Read the model definition and answer for the solid it produces. Units are mm, in the model's axes. A direction names the side the tool comes from. Coordinates: 2 decimals unless noted, no trailing zeros. Write each loop counter-clockwise with the first axis right and the second up, starting at its lowest first coordinate (ties: lowest second). Pieces come first, ordered by that corner, then holes. Notation, with made-up numbers: (76, 18.25) -> (100, 18.25) arc R31 ccw to (100, 56.25) -> close; hole circle Ø2 at (38.5, 15). An arc over 180 degrees is marked (long way). Use CSV: the item, a comma, the result in double quotes.
Autodesk Inventor part; units mm, degrees
ref_plane "YZ Plane" through (0, 0, 0) normal (1, 0, 0) x (0, 1, 0)
ref_plane "XZ Plane" through (0, 0, 0) normal (0, 1, 0) x (-1, 0, 0)
ref_plane "XY Plane" through (0, 0, 0) normal (0, 0, 1) x (1, 0, 0)
sketch "Sketch1" plane through (0, 0, 0) normal (0, 0, 1) x (1, 0, 0)
  line L0 (0, 0) -> (70, 0)
  line L1 (70, 0) -> (70, 77.5)
  line L2 (70, 77.5) -> (0, 77.5)
  line L3 (0, 77.5) -> (0, 0)
  dimension "d0" = 70
  dimension "d1" = 77.5
extrude "Extrusion1" add sketch "Sketch1" along normal blind 70
sketch "Sketch3" plane through (0, 0, 70) normal (0, 0, 1) x (1, 0, 0)
  line L0 (0, 0) -> (70, 0)
  line L1 (70, 77.5) -> (0, 77.5)
  line L2 (70, 0) -> (35, 0)
  line L3 (35, 0) -> (35, 77.5)
  line L4 (35, 77.5) -> (70, 77.5)
  line L5 (70, 77.5) -> (70, 0)
extrude "Extrusion3" cut sketch "Sketch3" against normal through all
sketch "Sketch4" plane through (0, 77.5, 70) normal (0, 1, 0) x (1, 0, 0)
  line L0 (0, 70) -> (0, 0)
  line L1 (0, 0) -> (-12.5, 0)
  line L2 (35, 70) -> (0, 70)
  arc A0 (-12.5, 0) -> (0, 70) centre (-1137.8005, 237.0626) ccw
  line L3 (-12.5, -10) -> (35, -10) construction
  dimension "d9" = 1150
  dimension "d54" = 47.5
  dimension "d55" = 10
extrude "Extrusion4" add sketch "Sketch4" against normal blind 77.5
sketch "Sketch5" plane through (35, 0, 70) normal (1, 0, 0) x (0, 0, -1)
  line L0 (0, 77.5) -> (0, 86.25)
  line L1 (0, 0) -> (0, -8.75)
  line L2 (0, 0) -> (0, 77.5)
  line L3 (70, 77.5) -> (70, 0)
  arc A0 (0, 86.25) -> (70, 77.5) centre (177.5728, 1222.4577) ccw
  arc A1 (70, 0) -> (0, -8.75) centre (177.5728, -1144.9577) ccw
  line L4 (0, 77.5) -> (70, 77.5)
  line L5 (70, 0) -> (0, 0)
  line L6 (-10, 86.25) -> (-10, -8.75) construction
  point P0 (-10, 38.75)
  point P1 (0, 38.75)
  dimension "d14" = 1150
  dimension "d15" = 1150
  dimension "d52" = 10
  dimension "d53" = 95
extrude "Extrusion5" add sketch "Sketch5" against normal blind 55 contours L0 A0 L4 | L5 A1 L1
sketch "Sketch6" plane through (-20, 0, 0) normal (0, 1, 0) x (1, 0, 0)
  line L0 (20, 0) -> (0, 0)
  line L1 (0, -70) -> (0, 0)
  arc A0 (7.5, -70) -> (20, 0) centre (-1117.8005, 167.0626) ccw
  line L2 (7.5, -70) -> (0, -70)
extrude "Extrusion6" cut sketch "Sketch6" along normal through all both and the other way through all
fillet "Fillet3" radius 19.35 2 edges at (-5.7463, 81.368, 35.3063) (-5.7463, -3.868, 35.3063)
sketch "Sketch8" plane through (0, 0, 70) normal (0, 0, 1) x (1, 0, 0)
  line L0 (35, 86.25) -> (35, -8.75)
  line L1 (35, 77.5) -> (35, 0)
  circle A0 centre (35, 38.75) radius 35
  point P0 (0, 0)
  dimension "d23" = 70
extrude "Extrusion7" cut sketch "Sketch8" against normal blind 17.5
sketch "Sketch17" plane through (35, 0, 0) normal (1, 0, 0) x (0, 0, -1)
  line L0 (-5, 13.75) -> (-40, 13.75)
  line L1 (-40, 13.75) -> (-40, 63.75)
  line L2 (-40, 63.75) -> (-5, 63.75)
  line L3 (-5, 63.75) -> (-5, 13.75)
  line L4 (0, 77.5) -> (0, 0)
  line L5 (-70, 86.25) -> (-70, 73.75)
  arc A0 (-70, 86.25) -> (0, 77.5) centre (107.5728, 1222.4577) ccw
  line L6 (-70, 3.75) -> (-70, 73.75)
  line L7 (-70, 3.75) -> (-70, -8.75)
  arc A1 (0, 0) -> (-70, -8.75) centre (107.5728, -1144.9577) ccw
  point P0 (-5, 38.75)
  point P1 (0, 38.75)
  dimension "d62" = 35
  dimension "d63" = 50
  dimension "d77" = 5
extrude "Extrusion15" cut sketch "Sketch17" against normal through all
sketch "Sketch21" plane through (35, 13.75, 5) normal (1, 0, 0) x (0, 0, -1)
  line L0 (-8, 5) -> (0, 5)
  line L1 (0, 5) -> (0, 45)
  line L2 (0, 45) -> (-8, 45)
  line L3 (-8, 45) -> (-8, 5)
  line L4 (0, 0) -> (0, 50)
  point P0 (5, -13.75)
  point P1 (-35, 25)
  point P2 (0, 25)
  dimension "d78" = 40
  dimension "d79" = 8
extrude "Extrusion19" cut sketch "Sketch21" against normal blind 30
sketch "Sketch22" plane through (35, 63.75, 40) normal (0, 1, 0) x (1, 0, 0)
  line L0 (0, 35) -> (0, 0)
  circle A0 centre (-15, 15) radius 2.5
  line L1 (0, 35) -> (-35.1041, 35)
  point P0 (-35, 40)
  dimension "d82" = 5
  dimension "d90" = 20
  dimension "d91" = 15
extrude "Extrusion20" cut sketch "Sketch22" against normal through all
sketch "Sketch23" plane through (35, 13.75, 40) normal (1, 0, 0) x (0, 0, -1)
  line L0 (35, 5) -> (27, 5) construction
  line L1 (27, 5) -> (27, 45) construction
  line L2 (27, 45) -> (35, 45) construction
  line L3 (35, 45) -> (35, 50) construction
  line L4 (35, 50) -> (0, 50) construction
  line L5 (0, 50) -> (0, 0) construction
  line L6 (0, 0) -> (35, 0) construction
  line L7 (35, 0) -> (35, 5) construction
  line L8 (35, 50) -> (0, 50)
  line L9 (0, 50) -> (35, 50)
  line L10 (35, 50) -> (35, 0)
  line L11 (35, 0) -> (0, 0)
  line L12 (0, 0) -> (0, 50)
  line L13 (34, 1) -> (34, 49)
  line L14 (34, 49) -> (1, 49)
  line L15 (1, 49) -> (1, 1)
  line L16 (1, 1) -> (34, 1)
  point P0 (40, -13.75)
  dimension "d86" = 1
extrude "Extrusion21" cut sketch "Sketch23" against normal through all
properties part number "AA016" material "ABS Plastic"
1. Find the intervals of material crossed by line 1 along Y through (x, z) = (8.5, 12.5); line 2 along Z through (x, y) = (20, 41); line 3 along X through (y, z) = (59, 27), in increasing order.
Solutions:
line 1,"y = 14.75 to 18.75, 58.75 to 62.75"
line 2,"z = 13 to 22.5, 27.5 to 39"
line 3,"x = -4.29 to 18.5, 21.5 to 35"
2. A cutting plane is placed at A-A (x = 20). Give the vertices of the cut face in (y, z).
Solutions:
outline,"(14.75, 6) -> (18.75, 6) -> (18.75, 13) -> (58.75, 13) -> (58.75, 6) -> (62.75, 6) -> (62.75, 22.5) -> (14.75, 22.5) -> close; (14.75, 27.5) -> (62.75, 27.5) -> (62.75, 39) -> (14.75, 39) -> close"
3. A cutting plane is placed at B-B (y = 28). Give the vertices of the cut face in (x, z), and give its area (3 significant figures).
Solutions:
outline,"(-6.41, 39) arc R1150 cw to (-0.9, 6) -> (5, 6) -> (5, 13) -> (35, 13) -> (35, 39) -> close; hole circle Ø5 at (20, 25)"
area,"1,040 mm^2"
4. A cutting plane is placed at C-C (x = 28). Give the vertices of the cut face in (y, z), and give its area (3 significant figures).
Solutions:
outline,"(14.75, 6) -> (18.75, 6) -> (18.75, 13) -> (58.75, 13) -> (58.75, 6) -> (62.75, 6) -> (62.75, 39) -> (14.75, 39) -> close"
area,"1,300 mm^2"
5. Each of these flat-tipped pins is pushed along its axis until it touches: pin 1 Ø1.5 at (y, z) = (57, 26.5) entering from -X; pin 2 Ø2 at (y, z) = (22, 35.5) entering from -X; pin 3 Ø4 at (x, y) = (30.5, 33) entering from -Z. Where does it stop, or does it pass through?
Solutions:
pin 1,"stops at x = -4.34"
pin 2,"stops at x = -5.96"
pin 3,"stops at z = 13"
6. For a pull along X with two mould halves and no side action, classify faces 1 (the cylindrical face through (18.16, 39.09, 23.31)), 2 (the flat face through (35, 38, 26)), 3 (the cylindrical face through (-3.574, 39.086, 22.751)), 4 (the flat face through (15, 39, 39)) as pulls with the +X half, pulls with the -X half, needs draft (parallel to the pull), parting line crosses it, or undercut.
Solutions:
face 1,"undercut"
face 2,"pulls with the +X half"
face 3,"pulls with the -X half"
face 4,"needs draft"
7. A tool of negligible diameter and unlimited length cuts with its end or side. For faces 5 (the flat face through (15, 14.75, 23)), 6 (the flat face through (20, 58.75, 9)), from which of +Z, -Z, +X, -X, +Y, -Y can it reach the whole face along a straight path? Write none if from no direction.
Solutions:
face 5,"+Z, -Z, +X, -X, -Y"
face 6,"-Z, +X"
